For this review, use the dimensioned drawing (mm, ordinates from the lowest corner) and the shaded views. Round coordinates to 2 decimals unless told otherwise and drop trailing zeros. Loops run counter-clockwise (first coordinate to the right, second up) from the corner with the lowest first, then second, coordinate; pieces in that order, holes last. Notation, with made-up numbers: (11.5, -1) - (56.5, -1) arc R9 ccw to (56.5, 16) - close; hole circle Ø6 at (8, -5). An arc over 180 degrees is marked (long way). Answer as CSV lines item,"result". Start each with the question number.
(1) Consider section C-C (x = 17). Give the boundary of the cut face in (y, z).
(2) Consider section A-A (z = 19.5). Give the boundary of the cut face in (x, y) (3 decimals).
(3) Mouldability with a two-part tool opening along X and no side actions: class the marked faces 1, 2, 3 and 4 as released by +X, released by -X, zero draft, split by the parting line, or undercut.
(4) Consider section B-B (x = 73.5). Give the boundary of the cut face in (y, z) (3 decimals).
(5) For P1, Ø3, axis at x = 56, z = 21.5, coming from the +Y side (3 decimals); P2, Ø1.6, axis at y = 23.5, z = 53, coming from the +X side, all flat-tipped, find the tip position at first contact; note any pin that passes through.
(6) Wall thickness on L1, parallel to Y at x = 32, z = 62 (3 decimals); L2, parallel to Y at x = 12, z = 61: over which ranges is each line inside the solid? List them lowest first.
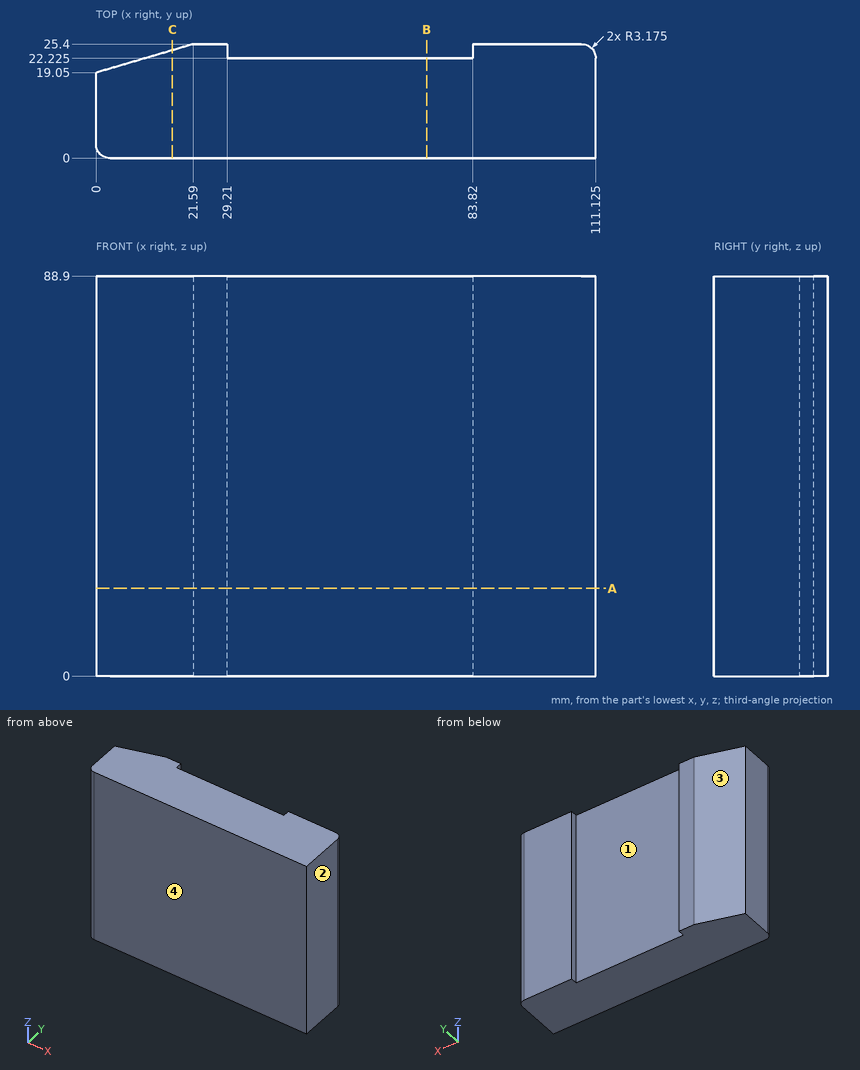
Determined:
1,outline,"(0, 0) - (24.05, 0) - (24.05, 88.9) - (0, 88.9) - close"
2,outline,"(0, 3.175) arc R3.175 ccw to (3.175, 0) - (111.125, 0) - (111.125, 22.225) arc R3.175 ccw to (107.95, 25.4) - (83.82, 25.4) - (83.82, 22.225) - (29.21, 22.225) - (29.21, 25.4) - (21.59, 25.4) - (0, 19.05) - close"
3,face 1,"undercut"
3,face 2,"released by +X"
3,face 3,"released by -X"
3,face 4,"zero draft"
4,outline,"(0, 0) - (22.225, 0) - (22.225, 88.9) - (0, 88.9) - close"
5,P1,"stops at y = 22.225"
5,P2,"stops at x = 111.09"
6,L1,"y = 0 to 22.225"
6,L2,"y = 0 to 22.58"
